The model under review builds one solid part; all positions refer to its coordinate system, in mm. Face numbers are marked on the shaded views. Give positions to 0.01 mm unless a question says otherwise; leave off trailing zeros. Write each loop counter-clockwise with the first axis right and the second up, starting at its lowest first coordinate (ties: lowest second). Pieces come first, ordered by that corner, then holes. Notation, with made-up numbers: (86.25, 53) - (113.25, 53) arc R14 ccw to (113.25, 80) - close; hole circle Ø8 at (1.25, 0). An arc over 180 degrees is marked (long way). Write item = value, one per line.
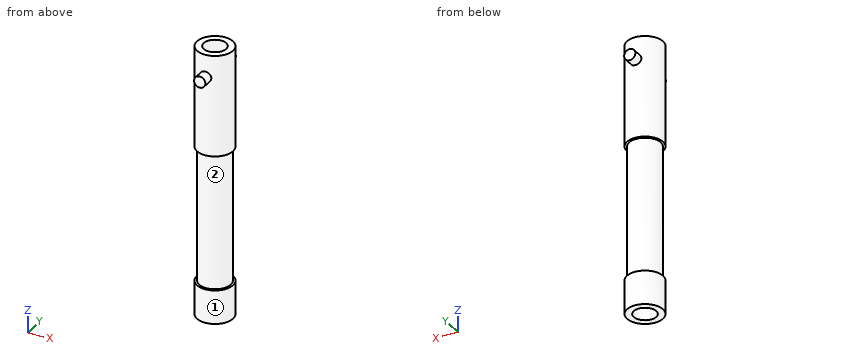
```python
from build123d import *

# Parameters (mm, degrees)
F2_R     = 2.5
F3_DEPTH = 12.5


with BuildPart() as f1:
    # F0 (on Front) → F1 (revolve)
    with BuildSketch(Plane.XZ):
        Polygon((8, 51), (5, 51), (5, -69), (8, -69), (8, -54), (7, -54), (7, 6), (8, 6), align=None)
    revolve(axis=Axis((0, 0, -22.5128643215), (0, 0, -1)))

    # F2 (on Front) → F3 (join, symmetric)
    with BuildSketch(Plane.XZ):
        with Locations((0, 41)):
            Circle(F2_R)
    extrude(amount=F3_DEPTH, both=True)


solid = f1.part
```
1. Take a section at B-B on x = 0. Give the boundary of the cut face in (y, z), and give its area (3 significant figures).
Findings below:
outline = (-12.5, 38.5) - (-8, 38.5) - (-8, 6) - (-7, 6) - (-7, -54) - (-8, -54) - (-8, -69) - (-5, -69) - (-5, 38.5) - (5, 38.5) - (5, -69) - (8, -69) - (8, -54) - (7, -54) - (7, 6) - (8, 6) - (8, 38.5) - (12.5, 38.5) - (12.5, 43.5) - (8, 43.5) - (8, 51) - (5, 51) - (5, 43.5) - (-5, 43.5) - (-5, 51) - (-8, 51) - (-8, 43.5) - (-12.5, 43.5) - close
area = 695 mm²
2. Take a section at A-A on y = 0. Give the boundary of the cut face in (x, z), and give its area (3 significant figures).
Findings below:
outline = (-8, -69) - (-5, -69) - (-5, 51) - (-8, 51) - (-8, 6) - (-7, 6) - (-7, -54) - (-8, -54) - close; circle Ø5 at (0, 41); (5, -69) - (8, -69) - (8, -54) - (7, -54) - (7, 6) - (8, 6) - (8, 51) - (5, 51) - close
area = 620 mm²
3. Draft analysis for pull direction Z (two halves, no side actions). For the marked faces 1 and 2, state which applies: +Z half, -Z half, draft (parallel to the pull), parting line (faces both ways), or undercut.
Findings below:
face_1 = draft
face_2 = undercut
4. Take a section at C-C on z = -7. Give the boundary of the cut face in (x, y), and give its area (3 significant figures).
Findings below:
outline = circle Ø14 at (0, 0); hole circle Ø10 at (0, 0)
area = 75.4 mm²
5. Insertion check: P1, Ø6, axis at x = 0, y = 0, coming from the -Z side; P2, Ø12, axis at y = -4, z = -5, coming from the +X side; P3, Ø2, axis at y = -2, z = 8, coming from the -X side; P4, Ø1, axis at y = 9.5, z = -56.5, coming from the +X side. Each pin has a flat end and moves straight along its axis. Give the tip position at first contact, or say it passes through.
Findings below:
P1 = 38.5
P2 = 7
P3 = -7.94
P4 = through
6. For line 1 (X direction, y = 0, z = -43.5); line 2 (Z direction, x = -5, y = -5), list the stretches that pass through material, from the lowest coordinate up. Write a range as from..to.
Findings below:
line_1 = -7..-5, 5..7
line_2 = -69..-54, 6..51
7. Take a section at D-D on z = 41. Give the boundary of the cut face in (x, y), and give its area (3 significant figures).
Findings below:
outline = (-2.5, -12.5) - (2.5, -12.5) - (2.5, -7.6) arc R8 ccw to (2.5, 7.6) - (2.5, 12.5) - (-2.5, 12.5) - (-2.5, 7.6) arc R8 ccw to (-2.5, -7.6) - close; hole (-2.5, -4.33) - (-2.5, 4.33) arc R5 ccw to start; hole (2.5, -4.33) arc R5 ccw to (2.5, 4.33) - close
area = 217 mm²
